from build123d import *

# Parameters (mm, degrees)
SKETCH1_W             = 100
SKETCH1_H             = 60
SKETCH1_R             = 1.13
BOSS_EXTRUDE1_DEPTH   = 4.7752
F_4_40_TAPPED_HOLE1_D = 2.2606


with BuildPart() as part:
    # Sketch1 → Boss-Extrude1 (new body)
    with BuildSketch(Plane.XY):
        with Locations((50, -30)):
            Rectangle(SKETCH1_W, SKETCH1_H)
        with Locations((15, -5)):
            Circle(SKETCH1_R, mode=Mode.SUBTRACT)
        with Locations((15, -55)):
            Circle(SKETCH1_R, mode=Mode.SUBTRACT)
        with Locations((85, -5)):
            Circle(SKETCH1_R, mode=Mode.SUBTRACT)
        with Locations((85, -55)):
            Circle(SKETCH1_R, mode=Mode.SUBTRACT)
    extrude(amount=BOSS_EXTRUDE1_DEPTH)

    # #4-40 Tapped Hole1 (through all)
    with Locations(Plane(origin=(15, -5, 4.7752), x_dir=(1, 0, 0), z_dir=(0, 0, 1))):
        with Locations((0, 0), (0, -50), (70, -50), (70, 0)):
            Hole(F_4_40_TAPPED_HOLE1_D / 2)


solid = part.part
Can you work these out from the model? Positions are in its coordinate system, mm. Give positions to 0.01 mm unless a question says otherwise; leave off trailing zeros. Order: outer loops, then holes, each group sorted by start corner. A loop starts at its lowest first (then second) coordinate and runs counter-clockwise, first axis right, second up. Notation, with made-up numbers: M -31.5,73.25 L 13.5,73.25 A25 cw 13.5,109.25 Z; hole C 69.25,13 d1. An arc over 180 degrees is marked long. Use a Markdown table: item, result. Add a question column.
Item 1: Suppose I cut it at B-B (y = -5). List the corners of the cut face in (x, z) for me, then the cut area to 3 significant figures.
Item 2: Suppose I cut it at A-A (x = 85). List the corners of the cut face in (y, z) for me.
Item 3: We'd pull the mould along X, two halves only. Please class faces 1 (the flat face through (100, -30, 2)), 2 (the flat face through (49, -30, 0)), 3 (the cylindrical face through (83.956, -5.433, 2.354)): +X half, -X half, draft (parallel to the pull), parting line (faces both ways), or undercut.
Item 4: Will this pin go through, and if not, where does the flat tip stop? pin 1 (1 mm diameter, centred on x = 67, z = 1, fed in from +Y).
Item 5: If I drill on L1, parallel to Y at x = 15, z = 3.1; L2, parallel to Y at x = 16, z = 4.15, over which ranges is the centre line in solid material (lowest first)? Write a range as [from, to].
Answer sheet:
| question | item | result |
|---|---|---|
| 1 | outline | M 0,0 L 13.87,0 L 13.87,4.78 L 0,4.78 Z; M 16.13,0 L 83.87,0 L 83.87,4.78 L 16.13,4.78 Z; M 86.13,0 L 100,0 L 100,4.78 L 86.13,4.78 Z |
| 1 | area | 456 mm² |
| 2 | outline | M -60,0 L -56.13,0 L -56.13,4.78 L -60,4.78 Z; M -53.87,0 L -6.13,0 L -6.13,4.78 L -53.87,4.78 Z; M -3.87,0 L 0,0 L 0,4.78 L -3.87,4.78 Z |
| 3 | face 1 | +X half |
| 3 | face 2 | draft |
| 3 | face 3 | undercut |
| 4 | pin 1 | stops at y = 0 |
| 5 | L1 | y = [-60, -56.13], [-53.87, -6.13], [-3.87, 0] |
| 5 | L2 | y = [-60, -55.53], [-54.47, -5.53], [-4.47, 0] |
